Read the model definition and answer for the solid it produces. Units are mm, in the model's axes. Face numbers are marked on the shaded views. A direction names the side the tool comes from. Give positions to 0.01 mm unless a question says otherwise; leave off trailing zeros. Loops run counter-clockwise (first coordinate to the right, second up) from the corner with the lowest first, then second, coordinate; pieces in that order, holes last.
(1) Straight lines are drawn through the part: probe 1 along X at (y, z) = (-3.5, 0); probe 2 along Z at (x, y) = (1.5, 9.5); probe 3 along Z at (x, y) = (1.75, -2.75). For each, find the intervals that lie inside material, in ascending order.
(2) Find section A-A, the plane z = 0. Write down the section's boundary in (x, y), then the cut area to 3 significant figures.
(3) Determine the mould class of the marked faces 1, 2 and 3 for opening direction X: pulls with the +X half, pulls with the -X half, needs draft (parallel to the pull), parting line crosses it, or undercut.
(4) Find section B-B, the plane y = 8.25. Write down the section's boundary in (x, z), then the cut area to 3 significant figures.
(5) Each of these flat-tipped pins is pushed along its axis until it touches: P1, Ø4, axis at y = 10, z = 3, coming from the +X side; P2, Ø4.5, axis at x = -1, z = 0.5, coming from the -Y side; P3, Ø5, axis at y = 3, z = -1.5, coming from the +X side; P4, Ø0.7, axis at y = -4, z = 0.5, coming from the +X side. Where does it stop, or does it pass through?
(6) Which of the six approach directions +Z, -Z, +X, -X, +Y, -Y give full straight-line access (tool end or side, diameter ignored) to the marked faces 4, 5 and 6?
```python
from build123d import *

# Parameters (mm, degrees)
SKETCH_1_R          = 4.25
EXTRUDE_1_DEPTH     = 5
SKETCH_2_R          = 2.5
EXTRUDE_2_DEPTH     = 12
CUT_EXTRUDE_START   = -5
CUT_EXTRUDE_1_DEPTH = 2.5
CHAMFER_1_SIZE      = 0.25


with BuildPart() as part:
    # 草图1 → 凸台-拉伸1 (new body)
    with BuildSketch(Plane(origin=(0, 0, 0), x_dir=(1, 0, 0), z_dir=(0, 1, 0))):
        with Locations(Location((0, 0, 0), (0, 0, 270))):
            Circle(SKETCH_1_R)
    extrude(amount=-EXTRUDE_1_DEPTH)

    # 草图2 → 凸台-拉伸2 (add)
    with BuildSketch(Plane(origin=(0, 0, 0), x_dir=(1, 0, 0), z_dir=(0, 1, 0))):
        with Locations(Location((0, 0, 0), (0, 0, 270))):
            Circle(SKETCH_2_R)
    extrude(amount=EXTRUDE_2_DEPTH)

    # 草图3 → 切除-拉伸1 (cut)
    with BuildSketch(Plane(origin=(0, 0, 0), x_dir=(1, 0, 0), z_dir=(0, 1, 0)).offset(CUT_EXTRUDE_START)):
        Polygon((2, -1.154700538), (2, 1.154700538), (0, 2.309401077), (-2, 1.154700538), (-2, -1.154700538), (0, -2.309401077), align=None)
    extrude(amount=CUT_EXTRUDE_1_DEPTH, mode=Mode.SUBTRACT)

    # 倒角1
    chamfer_1_edges = [part.edges().sort_by_distance(p)[0] for p in [
        (0, 0, -4.25),
        (0, -5, -4.25),
    ]]
    chamfer(chamfer_1_edges, length=CHAMFER_1_SIZE)


solid = part.part
```
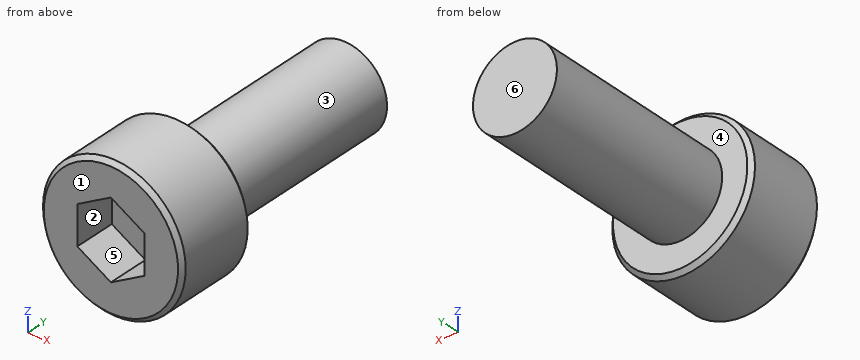
Entries:
1. probe 1: x = -4.25 to -2, 2 to 4.25
1. probe 2: z = -2 to 2
1. probe 3: z = -3.87 to -1.3, 1.3 to 3.87
2. outline: (-4.25, -4.75) - (-4, -5) - (-2, -5) - (-2, -2.5) - (2, -2.5) - (2, -5) - (4, -5) - (4.25, -4.75) - (4.25, -0.25) - (4, 0) - (2.5, 0) - (2.5, 12) - (-2.5, 12) - (-2.5, 0) - (-4, 0) - (-4.25, -0.25) - close
2. area: 92.4 mm2
3. face 1: needs draft
3. face 2: undercut
3. face 3: parting line crosses it
4. outline: circle Ø5 at (0, 0)
4. area: 19.6 mm2
5. P1: stops at x = 2.29
5. P2: stops at y = -5
5. P3: stops at x = 2.5
5. P4: stops at x = 4.25
6. face 4: +Y
6. face 5: -Y
6. face 6: +Z, -Z, +X, -X, +Y
